Could you check a few things on this model? Use its own coordinates, in mm. A direction names the side the tool comes from. Give positions to 0.01 mm unless a question says otherwise; leave off trailing zeros. Loops run counter-clockwise (first coordinate to the right, second up) from the corner with the lowest first, then second, coordinate; pieces in that order, holes last. Notation, with made-up numbers: (-10.5, 56) -> (30.5, 56) arc R21 ccw to (30.5, 95) -> close; hole circle Ø4 at (-29.75, -23.5). An arc over 180 degrees is marked (long way). Write each question's results on one line, items separated by ' | '. Start each with the question number.
Q1. Will these pins go through, and if not, where does the flat tip stop? P1, Ø10, axis at x = -8, y = 89.5, coming from the -Z side; P2, Ø1.5, axis at x = -17.5, y = 33, coming from the -Z side; P3, Ø5, axis at x = -19, y = 22, coming from the -Z side.
Q2. If we section it at A-A, the plane x = 0: List the corners of the cut face in (y, z) for me.
Q3. We'd pull the mould along Y, two halves only. Please class faces 3 (the face through (0.57, 101.01, 71.16)), 4 (the face through (0, 109.982, 1)), 5 (the face through (0, 18.03, 30)): released by +Y, released by -Y, zero draft, split by the parting line, or undercut.
Q4. If I drill on line 1 along Z through (x, y) = (0, 10.75); line 2 along Z through (x, y) = (0, 84); line 3 along Y through (x, z) = (11, 5), over which ranges is the centre line in solid material (lowest first)?
Q5. Which directions (+Z, -Z, +X, -X, +Y, -Y) give clear straight access to the entire face, cutting with the end or side of a thin tool? Please do faces 1 (the face through (0.57, 55.67, -5.97)), 2 (the face through (-2.18, 101.006, 35.548)).
Q6. If we section it at B-B, the plane z = 18.5: List the corners of the cut face in (x, y) for me, plus the area to 3 significant figures.
Q7. If we section it at D-D, the plane z = 40: List the corners of the cut face in (x, y) for me, plus the area to 3 significant figures.
Q8. If we section it at C-C, the plane y = 41: List the corners of the cut face in (x, z) for me.
from build123d import *

# Parameters (mm, degrees)
F0_R     = 9.962887
F0_R_2   = 10.057091
F1_DEPTH = 109.982
F2_W     = 74.247135
F2_H     = 110.230008
F3_DEPTH = 51.598741
F5_DEPTH = 79.502


with BuildPart() as f1:
    # F0 (on Front) → F1 (new body)
    with BuildSketch(Plane.XZ):
        with BuildLine():
            ThreePointArc((-25.79887, -45.365807), (0, -71.164677), (25.79887, -45.365807))
            Line((25.79887, -45.365807), (25.79887, 45.365807))
            ThreePointArc((25.79887, 45.365807), (0, 71.164677), (-25.79887, 45.365807))
            Line((-25.79887, 45.365807), (-25.79887, -45.365807))
        make_face()
        with Locations((0, -45.365807)):
            Circle(F0_R, mode=Mode.SUBTRACT)
        with Locations((0, 45.365807)):
            Circle(F0_R_2, mode=Mode.SUBTRACT)
    extrude(amount=-F1_DEPTH)

    # F2 (on face) → F3 (cut, through all)
    with BuildSketch(Plane.YZ.offset(25.79887)):
        with Locations((55.153735, 23.353766)):
            Rectangle(F2_W, F2_H)
    extrude(amount=-F3_DEPTH, mode=Mode.SUBTRACT)

    # F4 (on face) → F5 (join)
    with BuildSketch(Plane.XZ.offset(-92.277303)):
        with BuildLine():
            Line((-25.79887, -31.761238), (25.79887, -31.761238))
            ThreePointArc((25.79887, -31.761238), (0, -5.962368), (-25.79887, -31.761238))
        make_face()
    extrude(amount=F5_DEPTH)


solid = f1.part
Final values:
1) P1: stops at z = -70.99 | P2: stops at z = -64.99 | P3: stops at z = -65.2
2) outline: (0, -71.16) -> (109.98, -71.16) -> (109.98, -55.33) -> (0, -55.33) -> close; (0, -35.4) -> (109.98, -35.4) -> (109.98, 35.31) -> (92.28, 35.31) -> (92.28, -5.96) -> (18.03, -5.96) -> (18.03, 35.31) -> (0, 35.31) -> close; (0, 55.42) -> (18.03, 55.42) -> (18.03, 71.16) -> (0, 71.16) -> close; (92.28, 55.42) -> (109.98, 55.42) -> (109.98, 71.16) -> (92.28, 71.16) -> close
3) face 3: zero draft | face 4: released by +Y | face 5: undercut
4) line 1: z = -71.16 to -55.33, -35.4 to 35.31, 55.42 to 71.16 | line 2: z = -71.16 to -55.33, -35.4 to -5.96 | line 3: y = 0 to 18.03, 92.28 to 109.98
5) face 1: +Z | face 2: +Y, -Y
6) outline: (-25.8, 0) -> (25.8, 0) -> (25.8, 18.03) -> (-25.8, 18.03) -> close; (-25.8, 92.28) -> (25.8, 92.28) -> (25.8, 109.98) -> (-25.8, 109.98) -> close | area: 1,840 mm²
7) outline: (-25.8, 0) -> (-8.51, 0) -> (-8.51, 18.03) -> (-25.8, 18.03) -> close; (-25.8, 92.28) -> (-8.51, 92.28) -> (-8.51, 109.98) -> (-25.8, 109.98) -> close; (8.51, 0) -> (25.8, 0) -> (25.8, 18.03) -> (8.51, 18.03) -> close; (8.51, 92.28) -> (25.8, 92.28) -> (25.8, 109.98) -> (8.51, 109.98) -> close | area: 1,240 mm²
8) outline: (-25.8, -45.37) arc R25.8 ccw to (25.8, -45.37) -> (25.8, -31.76) arc R25.8 ccw to (-25.8, -31.76) -> close; hole circle Ø19.93 at (0, -45.37)
